Input: part model. Units: mm. Frame: model coordinates. Give positions to 0.01 mm unless a question says otherwise; leave off trailing zeros. Write each loop counter-clockwise with the first axis right and the second up, starting at its lowest first coordinate (ties: lowest second). Pieces come first, ordered by that corner, then holes. Notation, with made-up numbers: (0, -4) - (14, -4) arc R31 cw to (14, 31) - close; hole circle Ø10 at (40, -31). An arc over 180 degrees is marked (long way). Answer as CSV lines item,"result".
```python
from build123d import *

# Parameters (mm, degrees)
CUT_EXTRUDE1_START = -76.5048
SKETCH3_R          = 7.62
CUT_EXTRUDE1_DEPTH = 76.5048
SKETCH4_R          = 2.5527
CUT_EXTRUDE2_DEPTH = 76.5048
CHAMFER1_SIZE      = 0.508


with BuildPart() as part:
    # Sketch2 → Revolve1 (revolve)
    with BuildSketch(Plane(origin=(0, 0, 0), x_dir=(0, 0, -1), z_dir=(1, 0, 0)), mode=Mode.PRIVATE) as revolve1_sk:
        Polygon((1.27, 6.35), (1.27, 5.842), (2.2606, 5.842), (2.2606, 7.62), (74.2442, 7.62), (74.2442, 5.842), (75.2348, 5.842), (75.2348, 6.35), (76.5048, 6.35), (76.5048, 0), (0, 0), (0, 6.35), align=None)
    revolve(revolve1_sk.sketch.rotate(Axis((0, 0, 0), (0, 0, -1)), 90), axis=Axis((0, 0, 0), (0, 0, -1)))

    # Sketch3 → Cut-Extrude1 (cut)
    with BuildSketch(Plane.XY.offset(CUT_EXTRUDE1_START)):
        Circle(SKETCH3_R)
        with BuildLine():
            Line((6.816751826, 0.893039494), (4.181770802, 5.456960506))
            ThreePointArc((4.181770802, 5.456960506), (3.4375, 5.953924651), (2.634981025, 6.35))
            Line((2.634981025, 6.35), (-2.634981025, 6.35))
            ThreePointArc((-2.634981025, 6.35), (-3.4375, 5.953924651), (-4.181770802, 5.456960506))
            Line((-4.181770802, 5.456960506), (-6.816751826, 0.893039494))
            ThreePointArc((-6.816751826, 0.893039494), (-6.875, 0), (-6.816751826, -0.893039494))
            Line((-6.816751826, -0.893039494), (-4.181770802, -5.456960506))
            ThreePointArc((-4.181770802, -5.456960506), (-3.4375, -5.953924651), (-2.634981025, -6.35))
            Line((-2.634981025, -6.35), (2.634981025, -6.35))
            ThreePointArc((2.634981025, -6.35), (3.4375, -5.953924651), (4.181770802, -5.456960506))
            Line((4.181770802, -5.456960506), (6.816751826, -0.893039494))
            ThreePointArc((6.816751826, -0.893039494), (6.875, 0), (6.816751826, 0.893039494))
        make_face(mode=Mode.SUBTRACT)
    extrude(amount=CUT_EXTRUDE1_DEPTH, mode=Mode.SUBTRACT)

    # Sketch4 → Cut-Extrude2 (cut)
    with BuildSketch(Plane(origin=(0, 0, -76.5048), x_dir=(-1, 0, 0), z_dir=(0, 0, -1))):
        with Locations(Location((0, 0, 0), (0, 0, 90))):
            Circle(SKETCH4_R)
    extrude(amount=-CUT_EXTRUDE2_DEPTH, mode=Mode.SUBTRACT)

    # Chamfer1
    chamfer1_edges = [part.edges().sort_by_distance(p)[0] for p in [
        (-6.35, 0, 0),
        (-6.35, 0, -76.5048),
    ]]
    chamfer(chamfer1_edges, length=CHAMFER1_SIZE)


solid = part.part
```
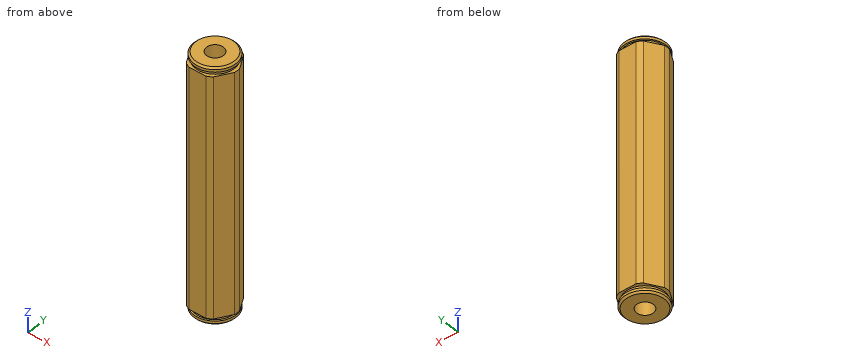
Item 1: Cut plane A-A on x = 0. Return the cut outline in (y, z), plus the area to 3 significant figures.
The answers:
outline,"(-6.35, -76) - (-5.84, -76.5) - (-2.55, -76.5) - (-2.55, 0) - (-5.84, 0) - (-6.35, -0.51) - (-6.35, -1.27) - (-5.84, -1.27) - (-5.84, -2.26) - (-6.35, -2.26) - (-6.35, -74.24) - (-5.84, -74.24) - (-5.84, -75.23) - (-6.35, -75.23) - close; (2.55, -76.5) - (5.84, -76.5) - (6.35, -76) - (6.35, -75.23) - (5.84, -75.23) - (5.84, -74.24) - (6.35, -74.24) - (6.35, -2.26) - (5.84, -2.26) - (5.84, -1.27) - (6.35, -1.27) - (6.35, -0.51) - (5.84, 0) - (2.55, 0) - close"
area,"578 mm²"
Item 2: Cut plane B-B on y = 0. Return the cut outline in (x, z) (3 decimals).
The answers:
outline,"(-6.875, -74.244) - (-5.842, -74.244) - (-5.842, -75.235) - (-6.35, -75.235) - (-6.35, -75.997) - (-5.842, -76.505) - (-2.553, -76.505) - (-2.553, 0) - (-5.842, 0) - (-6.35, -0.508) - (-6.35, -1.27) - (-5.842, -1.27) - (-5.842, -2.261) - (-6.875, -2.261) - close; (2.553, -76.505) - (5.842, -76.505) - (6.35, -75.997) - (6.35, -75.235) - (5.842, -75.235) - (5.842, -74.244) - (6.875, -74.244) - (6.875, -2.261) - (5.842, -2.261) - (5.842, -1.27) - (6.35, -1.27) - (6.35, -0.508) - (5.842, 0) - (2.553, 0) - close"
Item 3: Contact query for flat-ended pins moving along their axis: pin 1 (1.5 mm diameter, centred on y = 5, z = -24, fed in from -X); pin 2 (5 mm diameter, centred on y = -3, z = -65, fed in from +X); pin 3 (1.5 mm diameter, centred on y = 3.5, z = -67.5, fed in from -X). Output: stop coordinate, or through.
The answers:
pin 1,"x = -4.88"
pin 2,"x = 6.86"
pin 3,"x = -5.74"
Item 4: Ray query, line 1 (X direction, y = 0, z = -32) (3 decimals); line 2 (Z direction, x = 3, y = 5.5); line 3 (Y direction, x = -0.25, z = -16). Return the intervals inside material, ascending. Write a range as from..to.
The answers:
line 1,"-6.875..-2.553, 2.553..6.875"
line 2,"-76.08..-75.23, -74.24..-2.26, -1.27..-0.42"
line 3,"-6.35..-2.54, 2.54..6.35"
Item 5: Cut plane C-C on z = -42. Return the cut outline in (x, y) (3 decimals).
The answers:
outline,"(-6.817, -0.893) - (-4.182, -5.457) arc R6.875 ccw to (-2.635, -6.35) - (2.635, -6.35) arc R6.875 ccw to (4.182, -5.457) - (6.817, -0.893) arc R6.875 ccw to (6.817, 0.893) - (4.182, 5.457) arc R6.875 ccw to (2.635, 6.35) - (-2.635, 6.35) arc R6.875 ccw to (-4.182, 5.457) - (-6.817, 0.893) arc R6.875 ccw to start; hole circle Ø5.105 at (0, 0)"
